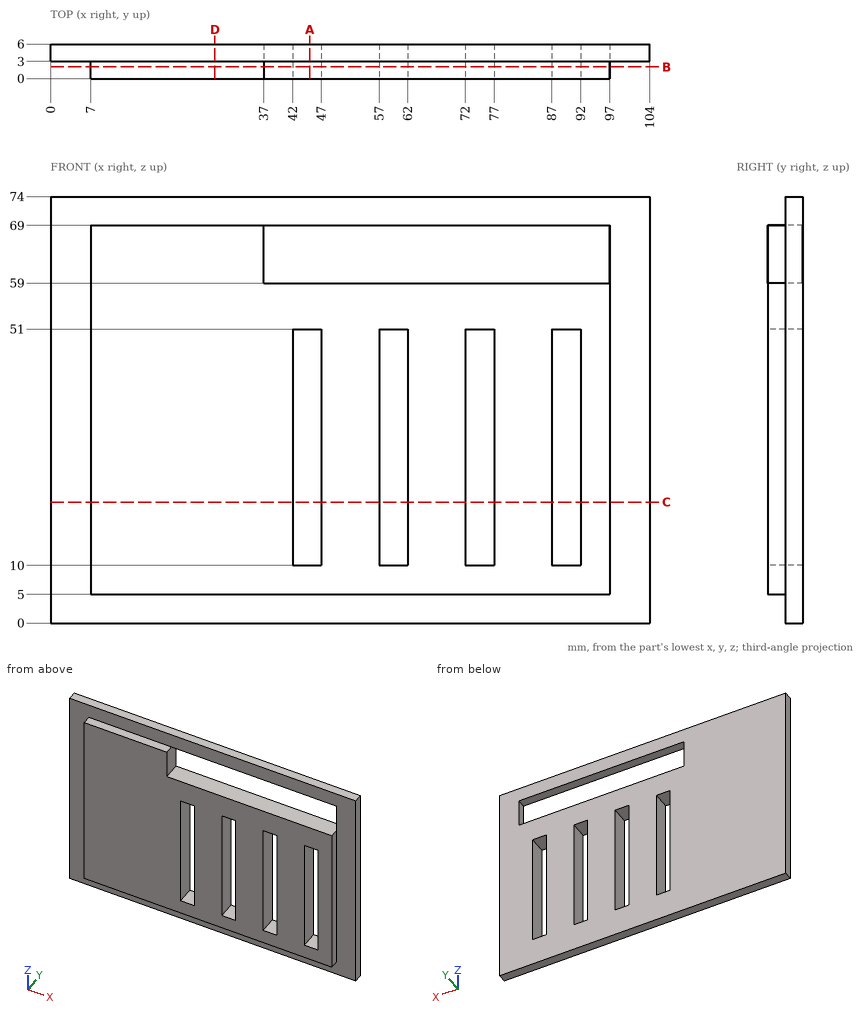
Source: three-view drawing plus pictorial views. Frame: mm from the lowest corner of the part. Round coordinates to 2 decimals unless told otherwise and drop trailing zeros. Loops run counter-clockwise (first coordinate to the right, second up) from the corner with the lowest first, then second, coordinate; pieces in that order, holes last.
Q1. Section B-B on y = 2.05. Return loops of the section in (x, z), plus the area to 3 significant figures.
Q2. Section D-D on x = 28.5. Return loops of the section in (y, z), plus the area to 3 significant figures.
Q3. Section A-A on x = 45. Return loops of the section in (y, z), plus the area to 3 significant figures.
Q4. Material intervals for L1, parallel to X at y = 4.05, z = 20; L2, parallel to Z at x = 45.5, y = 5.75; L3, parallel to X at y = 0.5, z = 30.5, sorted ascending.
Q5. Section C-C on z = 21. Return loops of the section in (x, y), plus the area to 3 significant figures.
Q6. Pin query (flat end, axial travel): P1, Ø2.5, axis at x = 25, y = 1.5, coming from the +Z side; P2, Ø1, axis at x = 89, y = 2, coming from the +Z side; P3, Ø2.5, axis at x = 38, y = 1.5, coming from the -Z side. Return the tip coordinate at first contact, or that it passes through.
Evaluation:
1. outline: (7, 5) - (97, 5) - (97, 59) - (37, 59) - (37, 69) - (7, 69) - close; hole (42, 10) - (47, 10) - (47, 51) - (42, 51) - close; hole (57, 10) - (62, 10) - (62, 51) - (57, 51) - close; hole (72, 10) - (77, 10) - (77, 51) - (72, 51) - close; hole (87, 10) - (92, 10) - (92, 51) - (87, 51) - close
1. area: 4,340 mm2
2. outline: (0, 5) - (3, 5) - (3, 0) - (6, 0) - (6, 74) - (3, 74) - (3, 69) - (0, 69) - close
2. area: 414 mm2
3. outline: (0, 5) - (3, 5) - (3, 0) - (6, 0) - (6, 10) - (0, 10) - close; (0, 51) - (6, 51) - (6, 59) - (0, 59) - close; (3, 69) - (6, 69) - (6, 74) - (3, 74) - close
3. area: 108 mm2
4. L1: x = 0 to 42, 47 to 57, 62 to 72, 77 to 87, 92 to 104
4. L2: z = 0 to 10, 51 to 59, 69 to 74
4. L3: x = 7 to 42, 47 to 57, 62 to 72, 77 to 87, 92 to 97
5. outline: (0, 3) - (7, 3) - (7, 0) - (42, 0) - (42, 6) - (0, 6) - close; (47, 0) - (57, 0) - (57, 6) - (47, 6) - close; (62, 0) - (72, 0) - (72, 6) - (62, 6) - close; (77, 0) - (87, 0) - (87, 6) - (77, 6) - close; (92, 0) - (97, 0) - (97, 3) - (104, 3) - (104, 6) - (92, 6) - close
5. area: 462 mm2
6. P1: stops at z = 69
6. P2: stops at z = 59
6. P3: stops at z = 5
